Geometry: final body of the model. Coordinates: model frame, mm. A direction names the side the tool comes from. Round coordinates to 2 decimals unless told otherwise and drop trailing zeros. Loops run counter-clockwise (first coordinate to the right, second up) from the corner with the lowest first, then second, coordinate; pieces in that order, holes last. Notation, with made-up numbers: (48.5, 86.5) - (78.5, 86.5) arc R23 ccw to (78.5, 113.5) - close; hole circle Ø3 at (65, 38.25). An arc over 180 degrees is marked (long way). Use CSV: the item, a comma, the result in double quotes.
from build123d import *

# Parameters (mm, degrees)
PAD_DEPTH           = 155
SKETCH001_R         = 2.5
SKETCH001_R_2       = 4.25
SKETCH001_R_3       = 3.45
SKETCH001_W         = 81.985035
SKETCH001_H         = 12
SKETCH001_W_2       = 6
POCKET_DEPTH        = 20
PAD001_DEPTH        = 6
SKETCH010_R         = 3.006811
SKETCH010_R_2       = 2.576879
PAD007_DEPTH        = 5.5
SKETCH011_W         = 6
SKETCH011_H         = 91
POCKET007_DEPTH     = 200
SKETCH012_R         = 1.875
POCKET008_DEPTH     = 200
SKETCH013_R         = 3.2
SKETCH013_R_2       = 0.1
PAD008_DEPTH        = 4
SKETCH014_R         = 5.2
SKETCH014_R_2       = 2.5
PAD009_DEPTH        = 8
PAD010_DEPTH        = 3
LINEARPATTERN_COUNT = 3
LINEARPATTERN_PITCH = 72.5
CHAMFER_SIZE2       = 3.8
CHAMFER_SIZE        = 2


with BuildPart() as part:
    # Sketch → Pad (new body)
    with BuildSketch(Plane.YZ):
        Polygon((-48.736008, 3), (46.263992, 3), (61.263992, -12), (61.263992, -97), (46.263992, -112), (-48.736008, -112), (-48.736008, -124), (46.263992, -124), (65.263992, -105), (65.263992, -4), (46.263992, 15), (-48.736008, 15), align=None)
    extrude(amount=-PAD_DEPTH)

    # Sketch001 (on Face9 of Pad) → Pocket (cut)
    with BuildSketch(Plane.ZX.offset(65.263992)):
        with Locations((-19, -20)):
            Circle(SKETCH001_R)
        with Locations((-19, -60)):
            Circle(SKETCH001_R)
        with Locations((-19, -100)):
            Circle(SKETCH001_R)
        with Locations((-47.23029, -60)):
            Circle(SKETCH001_R_2)
        with Locations((-47.23029, -90)):
            Circle(SKETCH001_R_2)
        with Locations((-84.23029, -60)):
            Circle(SKETCH001_R_3)
        with Locations((-84.23029, -90)):
            Circle(SKETCH001_R_3)
        with Locations((-76.007482, -16)):
            Rectangle(SKETCH001_W, SKETCH001_H)
        Polygon((-16.5, -123), (-16.5, -135), (-88.5, -135), (-88.5, -129), (-70.5, -129), (-70.5, -126), (-52.5, -126), (-52.5, -123), (-34.5, -123), align=None)
        with Locations((-87.23029, -41.973526)):
            Rectangle(SKETCH001_W_2, SKETCH001_H)
        with Locations((-87.23029, -108.026474)):
            Rectangle(SKETCH001_W_2, SKETCH001_H)
    extrude(amount=-POCKET_DEPTH, mode=Mode.SUBTRACT)

    # Sketch002 (on Face5 of Pocket) → Pad001 (join)
    with BuildSketch(Plane(origin=(-35, 0, 0), x_dir=(0, 1, 0), z_dir=(-1, 0, 0))):
        Polygon((61.263992, 56.149231), (61.263992, 97), (46.263992, 112), (1.263992, 112), (1.263992, 56.149231), align=None)
    extrude(amount=-PAD001_DEPTH)

    # Sketch010 (on Face5 of Pad001) → Pad007 (join)
    with BuildSketch(Plane(origin=(-136, 0, 0), x_dir=(0, 1, 0), z_dir=(-1, 0, 0))):
        Polygon((-17.423706, 64.031371), (61.263992, 76.63363), (61.263992, 33.370614), (-17.423706, 45.972874), align=None)
        with Locations((-5.011436, 55.002122)):
            Circle(SKETCH010_R, mode=Mode.SUBTRACT)
        with Locations((39.975639, 55.002122)):
            Circle(SKETCH010_R_2, mode=Mode.SUBTRACT)
    extrude(amount=PAD007_DEPTH)

    # Sketch011 (on Face2 of Pad007) → Pocket007 (cut)
    with BuildSketch(Plane(origin=(0, -48.736008, 0), x_dir=(0, 0, -1), z_dir=(0, -1, 0))):
        with Locations((-12, -77.5)):
            Rectangle(SKETCH011_W, SKETCH011_H)
        with Locations((121, -77.5)):
            Rectangle(SKETCH011_W, SKETCH011_H)
    extrude(amount=-POCKET007_DEPTH, mode=Mode.SUBTRACT)

    # Sketch012 (on Face8 of Pocket007) → Pocket008 (cut)
    with BuildSketch(Plane(origin=(0, 0, 9), x_dir=(0, -1, 0), z_dir=(0, 0, 1))):
        with Locations((-30.263992, -50)):
            Circle(SKETCH012_R)
        with Locations((29.736008, -50)):
            Circle(SKETCH012_R)
        with Locations((29.736008, -105)):
            Circle(SKETCH012_R)
        with Locations((-30.263992, -105)):
            Circle(SKETCH012_R)
    extrude(amount=-POCKET008_DEPTH, mode=Mode.SUBTRACT)

    # Sketch013 (on DatumPlane) → Pad008 (join)
    with BuildSketch(Plane.YX.offset(-3)):
        with Locations((34.904408, -145.100494)):
            Circle(SKETCH013_R)
        with Locations((34.904408, -145.100494)):
            Circle(SKETCH013_R_2, mode=Mode.SUBTRACT)
        with Locations((35.092834, -39.948879)):
            Circle(SKETCH013_R)
        with Locations((35.092834, -39.948879)):
            Circle(SKETCH013_R_2, mode=Mode.SUBTRACT)
        with Locations((-5.045681, -79.898949)):
            Circle(SKETCH013_R)
        with Locations((-5.045681, -79.898949)):
            Circle(SKETCH013_R_2, mode=Mode.SUBTRACT)
        with Locations((-40.19043, -145.100494)):
            Circle(SKETCH013_R)
        with Locations((-40.19043, -145.100494)):
            Circle(SKETCH013_R_2, mode=Mode.SUBTRACT)
        with Locations((-40.096222, -40.137306)):
            Circle(SKETCH013_R)
        with Locations((-40.096222, -40.137306)):
            Circle(SKETCH013_R_2, mode=Mode.SUBTRACT)
    extrude(amount=PAD008_DEPTH)

    # Sketch014 (on Face26 of Pad008) → Pad009 (join)
    with BuildSketch(Plane.ZX.offset(65.263992)):
        with Locations((-19, -20)):
            Circle(SKETCH014_R)
        with Locations((-19, -20)):
            Circle(SKETCH014_R_2, mode=Mode.SUBTRACT)
        with Locations((-19, -60)):
            Circle(SKETCH014_R)
        with Locations((-19, -60)):
            Circle(SKETCH014_R_2, mode=Mode.SUBTRACT)
        with Locations((-19, -100)):
            Circle(SKETCH014_R)
        with Locations((-19, -100)):
            Circle(SKETCH014_R_2, mode=Mode.SUBTRACT)
    extrude(amount=-PAD009_DEPTH)

    # Sketch015 (on DatumPlane) → Pad010 (join)
    with BuildSketch(Plane.YZ.offset(-4)):
        with BuildLine():
            ThreePointArc((46.952712, -112), (58.271814, -54.499966), (46.952367, 3))
            Line((61.263992, -12), (46.952367, 3))
            Line((61.263992, -12), (61.263992, -97.001692))
            Line((61.263992, -97.001692), (46.952712, -112))
        make_face()
    pad010 = extrude(amount=-PAD010_DEPTH)

    # LinearPattern: Pad010 ×3
    with Locations(*[(-i * LINEARPATTERN_PITCH, 0, 0) for i in range(1, LINEARPATTERN_COUNT)]):
        add(pad010)

    # Chamfer
    chamfer_edges = [part.edges().sort_by_distance(p)[0] for p in [
        (-40.137306, -43.296222, 3),
        (-79.898949, -8.245681, 3),
        (-145.100494, -43.39043, 3),
        (-145.100494, 31.704408, 3),
        (-39.948879, 31.892834, 3),
    ]]
    chamfer_side = part.faces().sort_by_distance((-77.361115, -1.220288, 3))[0]
    chamfer(chamfer_edges, length=CHAMFER_SIZE, length2=CHAMFER_SIZE2, reference=chamfer_side)


solid = part.part
Item 1: Section C-C on z = -38.5. Return the cut outline in (x, y), plus the area to 3 significant figures.
Final values:
outline,"(-155, 61.26) - (-152, 61.26) - (-152, 57.43) - (-149, 57.43) - (-149, 61.26) - (-141.5, 61.26) - (-141.5, 29.24) - (-136, 29.24) - (-136, 61.26) - (-135, 61.26) - (-135, 65.26) - (-155, 65.26) - close; (-123, 61.26) - (-79.5, 61.26) - (-79.5, 57.43) - (-76.5, 57.43) - (-76.5, 61.26) - (-22, 61.26) - (-22, 65.26) - (-123, 65.26) - close; (-10, 61.26) - (-7, 61.26) - (-7, 57.43) - (-4, 57.43) - (-4, 61.26) - (0, 61.26) - (0, 65.26) - (-10, 65.26) - close"
area,"735 mm²"
Item 2: Pin query (flat end, axial travel): P1, Ø2, axis at x = -50, y = -29.74, coming from the +Z side; P2, Ø5, axis at x = -32.5, y = 39.5, coming from the +Z side; P3, Ø10, axis at x = -106.5, z = -97.5, coming from the -Y side; P4, Ø0.9, axis at x = -127.5, y = 64, coming from the +Z side. Return the tip coordinate at first contact, or that it passes through.
Final values:
P1,"passes through"
P2,"stops at z = 15"
P3,"stops at y = 55.76"
P4,"stops at z = -2.29"
Item 3: Section B-B on y = -22. Return the cut outline in (x, z), plus the area to 3 significant figures.
Final values:
outline,"(-155, -124) - (-123, -124) - (-123, -118) - (-32, -118) - (-32, -124) - (0, -124) - (0, -112) - (-155, -112) - close; (-155, 3) - (0, 3) - (0, 15) - (-32, 15) - (-32, 9) - (-123, 9) - (-123, 15) - (-155, 15) - close"
area,"2,630 mm²"
Item 4: Material intervals for line 1 (Z direction, x = -81, y = -6); line 2 (Z direction, x = -23, y = -23); line 3 (X direction, y = 59.5, z = -57), sorted ascending.
Final values:
line 1,"z = -118 to -112, -1 to 9"
line 2,"z = -124 to -112, 3 to 15"
line 3,"x = -152 to -149, -141.5 to -136, -79.5 to -76.5, -35 to -29, -7 to -4"
Item 5: Section D-D on x = -60. Return the cut outline in (y, z), plus the area to 3 significant figures.
Final values:
outline,"(-48.74, -118) - (52.26, -118) - (65.26, -105) - (65.26, -87.68) - (61.26, -87.68) - (61.26, -97) - (46.26, -112) - (-48.74, -112) - close; (-48.74, 3) - (46.26, 3) - (61.26, -12) - (61.26, -13.8) - (57.26, -13.8) - (57.26, -16.5) - (65.26, -16.5) - (65.26, -4) - (52.26, 9) - (-48.74, 9) - close; (57.26, -24.2) - (61.26, -24.2) - (61.26, -42.98) - (65.26, -42.98) - (65.26, -21.5) - (57.26, -21.5) - close; (61.26, -80.78) - (65.26, -80.78) - (65.26, -51.48) - (61.26, -51.48) - close"
area,"1,820 mm²"
Item 6: Mould query, pull axis Y, two halves, no side actions, for faces 1 (the flat face through (0, 63, -54)), 2 (the flat face through (-94.16, 53.869, -104.395)), 3 (the conical face through (-142.872, -42.621, -0.615)). Classes: released by +Y, released by -Y, zero draft, split by the parting line, or undercut.
Final values:
face 1,"zero draft"
face 2,"released by -Y"
face 3,"undercut"
Item 7: Reachability of faces 4 (the flat face through (-40, -39, -1)), 5 (the flat face through (-7, 58.5, -54.2)), 6 (the flat face through (-152, 58.5, -54.2)), 7 (the flat face through (-2, 61.264, -54)), 8 (the cylindrical face through (-61.321, 63.292, -81.043)) from +Z, -Z, +X, -X, +Y, -Y: full face, straight path, thin tool, end or side. Return the list, or none.
Final values:
face 4,"+X, -X, -Y"
face 5,"-Y"
face 6,"-X, -Y"
face 7,"+X, -Y"
face 8,"+Y, -Y"
Item 8: Section A-A on x = -100. Return the cut outline in (y, z).
Final values:
outline,"(-48.74, -118) - (52.26, -118) - (65.26, -105) - (65.26, -21.5) - (57.26, -21.5) - (57.26, -24.2) - (61.26, -24.2) - (61.26, -97) - (46.26, -112) - (-48.74, -112) - close; (-48.74, 3) - (46.26, 3) - (61.26, -12) - (61.26, -13.8) - (57.26, -13.8) - (57.26, -16.5) - (65.26, -16.5) - (65.26, -4) - (52.26, 9) - (-48.74, 9) - close"
